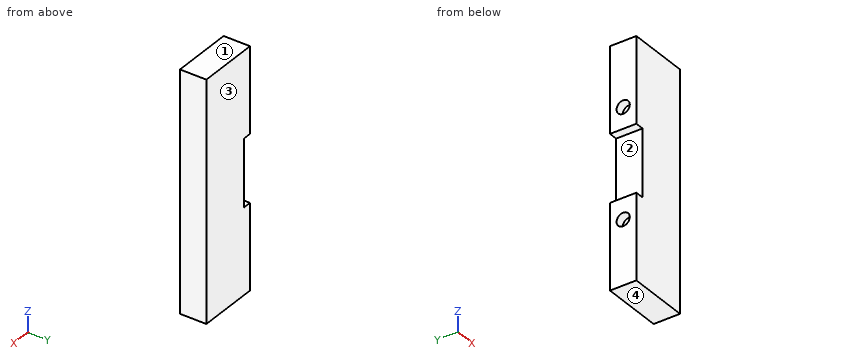
Autodesk Inventor part; units mm, degrees
ref_plane "YZ Plane" through (0, 0, 0) normal (1, 0, 0) x (0, 1, 0)
ref_plane "XZ Plane" through (0, 0, 0) normal (0, 1, 0) x (-1, 0, 0)
ref_plane "XY Plane" through (0, 0, 0) normal (0, 0, 1) x (1, 0, 0)
sketch "スケッチ1" plane through (0, 0, 0) normal (1, 0, 0) x (0, 1, 0)
  line L0 (0, 0) -> (5, 0)
  line L1 (5, 0) -> (5, -45)
  line L2 (5, -45) -> (0, -45)
  line L3 (0, -45) -> (0, 0)
  circle A0 centre (2.5, -12.15) radius 1.25
  line L4 (0, -13) -> (5, -13)
  line L5 (5, -13) -> (5, -32)
  line L6 (5, -32) -> (0, -32)
  line L7 (0, -32) -> (0, -13)
  circle A1 centre (2.5, -12.15) radius 3.5
  line L8 (0, -22.5) -> (5, -22.5)
  circle A2 centre (2.5, -32.85) radius 1.25
  line L9 (5, -16.15) -> (0, -16.15)
  line L10 (0, -16.15) -> (0, -28.85)
  line L11 (0, -28.85) -> (5, -28.85)
  line L12 (5, -28.85) -> (5, -16.15)
  point P0 (5, -28.85)
  point P1 (0, -28.85)
  point P2 (0, -16.15)
  point P3 (5, -16.15)
  dimension "d0" = 5
  dimension "d1" = 45
  dimension "d2" = 2.5
  dimension "d4" = 5
  dimension "d5" = 19
  dimension "d7" = 12.15
  dimension "d8" = 2.5
  dimension "d9" = 7
  dimension "d19" = 5
  dimension "d20" = 12.7
  dimension "d21" = 6.35
  dimension "d28" = 13
extrude "押し出し1" add sketch "スケッチ1" along normal blind 10 contours L0 L1 A1 L3 | A1 L1 L4 A0 L3 | L4 A0 L1 A1 L3 | A1 L1 L9 L3 | L4 A0 | A0 L4 | L9 L1 L8 L3 | L8 L1 L11 L3 | L11 L1 L6 A2 L3 | L6 A2 L1 L2 L3 | A2 L6 | L6 A2
extrude "押し出し2" add sketch "スケッチ1" against normal blind 1.651 contours L0 L1 A1 L3 | A1 L1 L4 A0 L3 | L4 A0 L1 A1 L3 | A1 L1 L9 L3 | L11 L1 L6 A2 L3 | L6 A2 L1 L2 L3
thread "ねじ1"
thread "ねじ2"
properties part number "belt_liner_v2_Plate_19" material "アルミニウム 6061"
Check sheet for the modelled part. Datum: model origin and axes. Units: mm. Face numbers are marked on the shaded views. Coordinates: 2 decimals unless noted, no trailing zeros. Order: outer loops, then holes, each group sorted by start corner. A loop starts at its lowest first (then second) coordinate and runs counter-clockwise, first axis right, second up. Notation, with made-up numbers: M 70,66 L 83,66 A32 cw 83,104 Z; hole C 82,61.5 d7. An arc over 180 degrees is marked long. Write each question's results on one line, items separated by ' | '. Start each with the question number.
1. Cross-section at C-C on z = -12.15. Record the cut outline in (x, y).
2. Cross-section at A-A on x = -1. Record the cut outline in (y, z).
3. Cross-section at D-D on y = 1.75. Record the cut outline in (x, z).
4. Material ranges on probe 1 along Z at (x, y) = (-1, 2.5); probe 2 along Y at (x, z) = (-0.4, -12.15); probe 3 along X at (y, z) = (2.1, -21), recorded low to high.
5. Cross-section at B-B on y = 4.6. Record the cut outline in (x, z).
6. Mould release check, pull along Z, two halves, no side actions. Record for the marked faces 1, 2, 3 and 4: +Z half, -Z half, draft (parallel to the pull), parting line (faces both ways), or undercut.
7. Go/stop test with a flat-tipped pin: P1, Ø2.5, axis at y = 2.5, z = -23, coming from the -X side. Record where the tip stops, or that it passes through.
Checks:
1) outline: M -1.65,0 L 10,0 L 10,5 L -1.65,5 L -1.65,3.75 L 0,3.75 L 0,1.25 L -1.65,1.25 Z
2) outline: M 0,-45 L 5,-45 L 5,-28.85 L 0,-28.85 Z; M 0,-16.15 L 5,-16.15 L 5,0 L 0,0 Z; hole C 2.5,-32.85 d2.5; hole C 2.5,-12.15 d2.5
3) outline: M -1.65,-45 L 10,-45 L 10,0 L -1.65,0 L -1.65,-11.15 L 0,-11.15 L 0,-13.15 L -1.65,-13.15 L -1.65,-16.15 L 0,-16.15 L 0,-28.85 L -1.65,-28.85 L -1.65,-31.85 L 0,-31.85 L 0,-33.85 L -1.65,-33.85 Z
4) probe 1: z = -45 to -34.1, -31.6 to -28.85, -16.15 to -13.4, -10.9 to 0 | probe 2: y = 0 to 1.25, 3.75 to 5 | probe 3: x = 0 to 10
5) outline: M -1.65,-45 L 10,-45 L 10,0 L -1.65,0 L -1.65,-16.15 L 0,-16.15 L 0,-28.85 L -1.65,-28.85 Z
6) face 1: +Z half | face 2: undercut | face 3: draft | face 4: -Z half
7) P1: stops at x = 0
